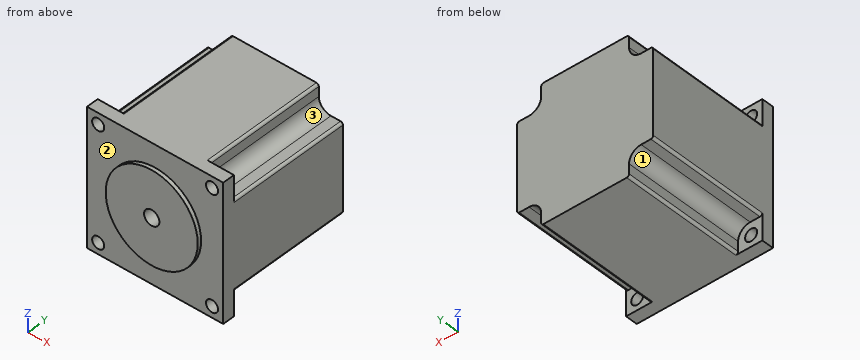
from build123d import *

# Parameters (mm, degrees)
F0_W     = 56.4
F0_H     = 56.4
F0_R     = 2.5
F1_DEPTH = 5
F3_DEPTH = 51
F4_R     = 5
F5_R     = 1
F6_R     = 19.05
F7_DEPTH = 1.6
F8_R     = 3.175
F9_DEPTH = 25


with BuildPart() as f1:
    # F0 (on Front) → F1 (new body)
    with BuildSketch(Plane.XZ):
        Rectangle(F0_W, F0_H)
        with Locations((-23.57, -23.57)):
            Circle(F0_R, mode=Mode.SUBTRACT)
        with Locations((23.57, -23.57)):
            Circle(F0_R, mode=Mode.SUBTRACT)
        with Locations((-23.57, 23.57)):
            Circle(F0_R, mode=Mode.SUBTRACT)
        with Locations((23.57, 23.57)):
            Circle(F0_R, mode=Mode.SUBTRACT)
    extrude(amount=F1_DEPTH)

    # F2 (on face) → F3 (join)
    with BuildSketch(Plane(origin=(0, 0, 0), x_dir=(-1, 0, 0), z_dir=(0, 1, 0))):
        Polygon((18.2, 18.2), (18.2, 28.2), (0, 28.2), (-18.2, 28.2), (-18.2, 18.2), (-28.2, 18.2), (-28.2, 0), (-28.2, -18.2), (-18.2, -18.2), (-18.2, -28.2), (0, -28.2), (18.2, -28.2), (18.2, -18.2), (28.2, -18.2), (28.2, 0), (28.2, 18.2), align=None)
    extrude(amount=F3_DEPTH)

    # F4
    f4_edges = [f1.edges().sort_by_distance(p)[0] for p in [
        (18.2, 25.5, 18.2),
        (18.2, 25.5, -18.2),
        (-18.2, 25.5, -18.2),
        (-18.2, 25.5, 18.2),
    ]]
    fillet(f4_edges, radius=F4_R)

    # F5
    f5_edges = [f1.edges().sort_by_distance(p)[0] for p in [
        (28.2, 25.5, 18.2),
        (18.2, 25.5, 28.2),
        (-18.2, 25.5, 28.2),
        (28.2, 25.5, -18.2),
        (18.2, 25.5, -28.2),
        (-18.2, 25.5, -28.2),
        (-28.2, 25.5, -18.2),
        (-28.2, 25.5, 18.2),
    ]]
    fillet(f5_edges, radius=F5_R)

    # F6 (on face) → F7 (join)
    with BuildSketch(Plane.XZ.offset(5)):
        Circle(F6_R)
    extrude(amount=F7_DEPTH)

    # F8 (on face) → F9 (cut)
    with BuildSketch(Plane.XZ.offset(6.6)):
        Circle(F8_R)
    extrude(amount=-F9_DEPTH, mode=Mode.SUBTRACT)


solid = f1.part
Here's how the part is built. I have some questions about the finished solid (model axes, mm). Face numbers are marked on the shaded views. A direction names the side the tool comes from. Give positions to 0.01 mm unless a question says otherwise; leave off trailing zeros. Loops run counter-clockwise (first coordinate to the right, second up) from the corner with the lowest first, then second, coordinate; pieces in that order, holes last. Notation, with made-up numbers: (81.25, -11.75) -> (117.25, -11.75) arc R18 cw to (117.25, 3.25) -> close; hole circle Ø10 at (50, -9). An arc over 180 degrees is marked (long way). Answer as a JSON object with one key per item and string values. Group by question number.
Item 1: I need wall thicknesses on L1, parallel to Z at x = -23.57, y = -3.4; L2, parallel to X at y = -3, z = 23; L3, parallel to Y at x = 16, z = -18.5. Which ranges of each line are inside material? Lowest first, please.
Item 2: Will these pins go through, and if not, where does the flat tip stop? pin 1 (2 mm diameter, centred on x = -25, y = 31.5, fed in from +Z); pin 2 (3 mm diameter, centred on y = 29.5, z = 25, fed in from +X); pin 3 (5 mm diameter, centred on x = 20, y = 4.5, fed in from +Z).
Item 3: Imagine slicing it at C-C on x = -2. Write out the boundary of the cut face in (y, z).
Item 4: Imagine slicing it at D-D on y = 41. Write out the boundary of the cut face in (x, z), then the cut area to 3 significant figures.
Item 5: On a 3-axis mill with a long thin cutter (end or side, diameter ignored), from which of +Z, -Z, +X, -X, +Y, -Y can I reach the whole of each face in a straight line? I mean the marked faces 1, 2 and 3. Say none if no direction works.
Item 6: Imagine slicing it at A-A on y = 17.5. Write out the boundary of the cut face in (x, z) (3 decimals).
Item 7: Imagine slicing it at B-B on z = 0. Write out the boundary of the cut face in (x, y) (3 decimals).
Answer list:
{
 "1": {"L1": "z = -28.2 to -26.07, -21.07 to 21.07, 26.07 to 28.2", "L2": "x = -28.2 to -26, -21.14 to 21.14, 26 to 28.2", "L3": "y = -5 to 51"},
 "2": {"pin 1": "stops at z = 18.2", "pin 2": "stops at x = 18.2", "pin 3": "stops at z = 28.15"},
 "3": {"outline": "(-6.6, -18.94) -> (-5, -18.94) -> (-5, -28.2) -> (51, -28.2) -> (51, 28.2) -> (-5, 28.2) -> (-5, 18.94) -> (-6.6, 18.94) -> (-6.6, 2.47) -> (18.4, 2.47) -> (18.4, -2.47) -> (-6.6, -2.47) -> close"},
 "4": {"outline": "(-28.2, -17.2) arc R1 ccw to (-27.2, -18.2) -> (-23.2, -18.2) arc R5 cw to (-18.2, -23.2) -> (-18.2, -27.2) arc R1 ccw to (-17.2, -28.2) -> (17.2, -28.2) arc R1 ccw to (18.2, -27.2) -> (18.2, -23.2) arc R5 cw to (23.2, -18.2) -> (27.2, -18.2) arc R1 ccw to (28.2, -17.2) -> (28.2, 17.2) arc R1 ccw to (27.2, 18.2) -> (23.2, 18.2) arc R5 cw to (18.2, 23.2) -> (18.2, 27.2) arc R1 ccw to (17.2, 28.2) -> (-17.2, 28.2) arc R1 ccw to (-18.2, 27.2) -> (-18.2, 23.2) arc R5 cw to (-23.2, 18.2) -> (-27.2, 18.2) arc R1 ccw to (-28.2, 17.2) -> close", "area": "2,800 mm2"},
 "5": {"face 1": "-Z, -X, +Y", "face 2": "-Y", "face 3": "+Z, +X, +Y"},
 "6": {"outline": "(-28.2, -17.2) arc R1 ccw to (-27.2, -18.2) -> (-23.2, -18.2) arc R5 cw to (-18.2, -23.2) -> (-18.2, -27.2) arc R1 ccw to (-17.2, -28.2) -> (17.2, -28.2) arc R1 ccw to (18.2, -27.2) -> (18.2, -23.2) arc R5 cw to (23.2, -18.2) -> (27.2, -18.2) arc R1 ccw to (28.2, -17.2) -> (28.2, 17.2) arc R1 ccw to (27.2, 18.2) -> (23.2, 18.2) arc R5 cw to (18.2, 23.2) -> (18.2, 27.2) arc R1 ccw to (17.2, 28.2) -> (-17.2, 28.2) arc R1 ccw to (-18.2, 27.2) -> (-18.2, 23.2) arc R5 cw to (-23.2, 18.2) -> (-27.2, 18.2) arc R1 ccw to (-28.2, 17.2) -> close; hole circle Ø6.35 at (0, 0)"},
 "7": {"outline": "(-28.2, -5) -> (-19.05, -5) -> (-19.05, -6.6) -> (-3.175, -6.6) -> (-3.175, 18.4) -> (3.175, 18.4) -> (3.175, -6.6) -> (19.05, -6.6) -> (19.05, -5) -> (28.2, -5) -> (28.2, 51) -> (-28.2, 51) -> close"}
}
